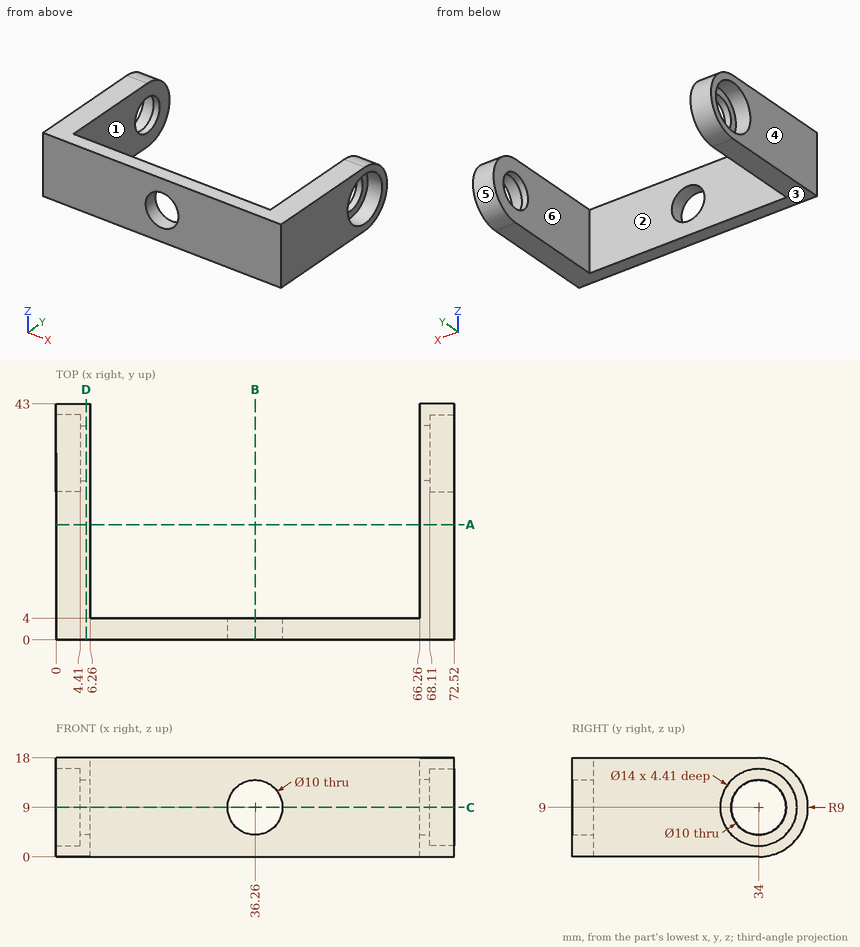
Could you check a few things on this drawing? It's one solid part, dimensions in mm from its lowest x, y, z. A direction names the side the tool comes from. Coordinates: 2 decimals unless noted, no trailing zeros. Loops run counter-clockwise (first coordinate to the right, second up) from the corner with the lowest first, then second, coordinate; pieces in that order, holes last. Notation, with made-up numbers: (84, -2) - (134, -2) arc R15 ccw to (134, 23) - close; hole circle Ø6 at (19, -17). An arc over 180 degrees is marked (long way). Return JSON: item names as keys, results as strings. Group by question number.
Item 1: If we section it at C-C on z = 9: Write out the boundary of the cut face in (x, y), and give its area (3 significant figures).
Item 2: If we section it at B-B on x = 36.26: Write out the boundary of the cut face in (y, z).
Item 3: If we section it at A-A on y = 21: Write out the boundary of the cut face in (x, z).
Item 4: On a 3-axis mill with a long thin cutter (end or side, diameter ignored), from which of +Z, -Z, +X, -X, +Y, -Y can I reach the whole of each face in a straight line? I mean the marked faces 5 and 6. Say none if no direction works.
Item 5: If we section it at D-D on x = 5.5: Write out the boundary of the cut face in (y, z), and give its area (3 significant figures).
Item 6: We'd pull the mould along X, two halves only. Please class the marked faces 1, 2, 3 and 4: +X half, -X half, draft (parallel to the pull), parting line (faces both ways), or undercut.
Item 7: I need wall thicknesses on line 1 (Y direction, x = 67.6, z = 9); line 2 (Z direction, x = 36.26, y = 2.7); line 3 (X direction, y = 1.8, z = 9). Which ranges of each line are inside material? Lowest first, please. Write a range as from..to.
Item 8: Will these pins go through, and if not, where does the flat tip stop? P1, Ø6, axis at x = 58, z = 7.5, coming from the +Y side; P2, Ø7, axis at y = 31.5, z = 11, coming from the -X side.
Calculated:
{
 "1": {"outline": "(0, 0) - (31.26, 0) - (31.26, 4) - (6.26, 4) - (6.26, 29) - (4.41, 29) - (4.41, 27) - (0, 27) - close; (0, 41) - (4.41, 41) - (4.41, 39) - (6.26, 39) - (6.26, 43) - (0, 43) - close; (41.26, 0) - (72.52, 0) - (72.52, 27) - (68.11, 27) - (68.11, 29) - (66.26, 29) - (66.26, 4) - (41.26, 4) - close; (66.26, 39) - (68.11, 39) - (68.11, 41) - (72.52, 41) - (72.52, 43) - (66.26, 43) - close", "area": "578 mm^2"},
 "2": {"outline": "(0, 0) - (4, 0) - (4, 4) - (0, 4) - close; (0, 14) - (4, 14) - (4, 18) - (0, 18) - close"},
 "3": {"outline": "(0, 0) - (6.26, 0) - (6.26, 18) - (0, 18) - close; (66.26, 0) - (72.52, 0) - (72.52, 18) - (66.26, 18) - close"},
 "4": {"face 5": "+X, -X, +Y", "face 6": "+Z, -Z, +Y"},
 "5": {"outline": "(0, 0) - (34, 0) arc R9 ccw to (34, 18) - (0, 18) - close; hole circle Ø10 at (34, 9)", "area": "661 mm^2"},
 "6": {"face 1": "undercut", "face 2": "undercut", "face 3": "draft", "face 4": "-X half"},
 "7": {"line 1": "y = 0..29, 39..43", "line 2": "z = 0..4, 14..18", "line 3": "x = 0..31.26, 41.26..72.52"},
 "8": {"P1": "stops at y = 4", "P2": "stops at x = 4.41"}
}
